from build123d import *

# Parameters (mm, degrees)
F0_R     = 25.5016
F1_DEPTH = 11.303
F2_R     = 22.7965
F5_DEPTH = 34.6022074724
F4_W     = 22.6323335914
F4_H     = 8.255


with BuildPart() as f1:
    # F0 (on Front) → F1 (new body)
    with BuildSketch(Plane.XZ):
        Circle(F0_R)
    extrude(amount=-F1_DEPTH)

    # F2 (on face) → F5 (join, through all)
    with BuildSketch(Plane(origin=(0, 11.303, 0), x_dir=(-1, 0, 0), z_dir=(0, 1, 0))):
        Circle(F2_R)
    extrude(amount=F5_DEPTH)

    # F4 (on Right) → F6 (revolve, cut)
    with BuildSketch(Plane.YZ):
        Polygon((0, 21.6916), (0, 0), (23.272873881, 0), (23.272873881, 8.255), align=None)
        with Locations((34.5890406767, 4.1275)):
            Rectangle(F4_W, F4_H)
        Polygon((45.9052074724, 12.65428), (23.272873881, 8.255), (45.9052074724, 8.255), align=None)
    revolve(axis=Axis((0, 11.6364369405, 0), (0, 1, 0)), mode=Mode.SUBTRACT)


solid = f1.part
Input: part model. Units: mm. Frame: model coordinates. A direction names the side the tool comes from. Coordinates: 2 decimals unless noted, no trailing zeros. Loops run counter-clockwise (first coordinate to the right, second up) from the corner with the lowest first, then second, coordinate; pieces in that order, holes last. Notation, with made-up numbers: (82, 21) - (124, 21) arc R34 cw to (124, 51) - close; hole circle Ø9 at (28, 10). An arc over 180 degrees is marked (long way). Answer in a Markdown table with one row per item. Add a question column.
Item 1: Contact query for flat-ended pins moving along their axis: P1, Ø2, axis at x = -2, z = 20, coming from the -Y side; P2, Ø4, axis at x = -5, z = -14.5, coming from the -Y side; P3, Ø8, axis at x = 16, y = 31, coming from the -Z side. Output: stop coordinate, or through.
Item 2: Section query C-C on y = 25. Return the cut outline in (x, z).
Item 3: Line query: line 1 along Y through (x, z) = (17, 15.5); line 2 along Z through (x, y) = (-8, 35.5); line 3 along Z through (x, y) = (-5.5, 2). Output: solid intervals per line, ascending. Write a range as [from, to].
Item 4: Access query for faces 4 (the flat face through (-19, 11.303, -13)), 5 (the flat face through (7, 0, 21)). Directions: +Z, -Z, +X, -X, +Y, -Y. A direction counts if a zero-diameter tool reaches every point of the face in a straight line with its end or side. Return the directions, or none.
Item 5: Section query B-B on z = 0. Return the cut outline in (x, y) (1 decimal).
Item 6: Section query A-A on x = 0. Return the cut outline in (y, z) (1 decimal), then the cut area to 3 significant figures.
Item 7: Section query D-D on y = 12.5. Return the cut outline in (x, z).
Item 8: Mould query, pull axis Z, two halves, no side actions, for faces 1 (the flat face through (-10, 45.905, -10)), 2 (the conical face through (-9.7, 31.92, -2.15)), 3 (the cylindrical face through (4.942, 28.362, -22.254)). Classes: released by +Z, released by -Z, zero draft, split by the parting line, or undercut.
Recorded:
| question | item | result |
|---|---|---|
| 1 | P1 | y = 1.03 |
| 1 | P2 | y = 7.54 |
| 1 | P3 | z = -19.38 |
| 2 | outline | circle Ø45.59 at (0, 0); hole circle Ø17.18 at (0, 0) |
| 3 | line 1 | [0, 11.3] |
| 3 | line 2 | [-21.35, -7], [7, 21.35] |
| 3 | line 3 | [-24.9, -19.79], [19.79, 24.9] |
| 4 | face 4 | +Y |
| 4 | face 5 | +Z, -Z, +X, -X, -Y |
| 5 | outline | (-25.5, 0) - (-21.7, 0) - (-8.3, 23.3) - (-12.7, 45.9) - (-22.8, 45.9) - (-22.8, 11.3) - (-25.5, 11.3) - close; (8.3, 23.3) - (21.7, 0) - (25.5, 0) - (25.5, 11.3) - (22.8, 11.3) - (22.8, 45.9) - (12.7, 45.9) - close |
| 6 | outline | (0, -25.5) - (11.3, -25.5) - (11.3, -22.8) - (45.9, -22.8) - (45.9, -12.7) - (23.3, -8.3) - (0, -21.7) - close; (0, 21.7) - (23.3, 8.3) - (45.9, 12.7) - (45.9, 22.8) - (11.3, 22.8) - (11.3, 25.5) - (0, 25.5) - close |
| 6 | area | 984 mm^2 |
| 7 | outline | circle Ø45.59 at (0, 0); hole circle Ø28.95 at (0, 0) |
| 8 | face 1 | zero draft |
| 8 | face 2 | undercut |
| 8 | face 3 | split by the parting line |
